```python
from build123d import *

# Parameters (mm, degrees)
SKETCH_2_R          = 1
CUT_EXTRUDE_1_DEPTH = 10
SKETCH_3_R          = 2.5
CUT_EXTRUDE_2_DEPTH = 2.5


with BuildPart() as part:
    # 草图1 → 旋转1 (revolve)
    with BuildSketch(Plane.XY, mode=Mode.PRIVATE) as revolve_1_sk:
        Polygon((0, 26), (3, 26), (3, 6), (9.5, 6), (10, 5.5), (10, 0), (3, 0), (3, 3), (0, 3), align=None)
    revolve(revolve_1_sk.sketch.rotate(Axis((0, 9.947317903, 0), (0, -1, 0)), 90), axis=Axis((0, 9.947317903, 0), (0, -1, 0)))

    # 草图2 → 切除-拉伸1 (cut)
    with BuildSketch(Plane(origin=(0, 6, 0), x_dir=(1, 0, 0), z_dir=(0, 1, 0))):
        with Locations(Location((0, 6, 0), (0, 0, 270))):
            Circle(SKETCH_2_R)
        with Locations(Location((6, 0, 0), (0, 0, 270))):
            Circle(SKETCH_2_R)
        with Locations(Location((0, -6, 0), (0, 0, 270))):
            Circle(SKETCH_2_R)
        with Locations(Location((-6, 0, 0), (0, 0, 270))):
            Circle(SKETCH_2_R)
    extrude(amount=-CUT_EXTRUDE_1_DEPTH, mode=Mode.SUBTRACT)

    # 草图3 → 切除-拉伸2 (cut)
    with BuildSketch(Plane(origin=(0, 6, 0), x_dir=(1, 0, 0), z_dir=(0, 1, 0))):
        with Locations(Location((0, 6, 0), (0, 0, 270))):
            Circle(SKETCH_3_R)
        with Locations(Location((6, 0, 0), (0, 0, 270))):
            Circle(SKETCH_3_R)
        with Locations(Location((0, -6, 0), (0, 0, 270))):
            Circle(SKETCH_3_R)
        with Locations(Location((-6, 0, 0), (0, 0, 270))):
            Circle(SKETCH_3_R)
    extrude(amount=-CUT_EXTRUDE_2_DEPTH, mode=Mode.SUBTRACT)


solid = part.part
```
Geometry: final body of the model. Coordinates: model frame, mm. A direction names the side the tool comes from. Round coordinates to 2 decimals unless told otherwise and drop trailing zeros. Order: outer loops, then holes, each group sorted by start corner. A loop starts at its lowest first (then second) coordinate and runs counter-clockwise, first axis right, second up. Notation, with made-up numbers: (21, -0.5) -> (71, -0.5) arc R16 ccw to (71, 12.5) -> close; hole circle Ø7 at (67, -20.75). An arc over 180 degrees is marked (long way). Use CSV: the item, a comma, the result in double quotes. Start each with the question number.
1) Set-up query: faces 4 (the face through (-0.6, 1.8, -6.8)), 5 (the face through (0, 3, 0)), 6 (the face through (0.751, 4.768, -3.615)). Return all of +Z, -Z, +X, -X, +Y, -Y with unobstructed straight access to the full face (end or side cutting, diameter ignored); none if empty.
2) Section C-C (y = 1.5). Return the cut outline in (x, z), and give its area (3 significant figures).
3) Section D-D (y = 20.75). Return the cut outline in (x, z), and give its area (3 significant figures).
4) Section A-A (x = 0). State how many separate pieces and enclosed holes the cut face has, and give its area (3 significant figures).
5) Draft query along X for faces 1 (the face through (-0.9, 15.86, 2.86)), 2 (the face through (0.751, 4.768, 8.385)), 3 (the face through (-2.4, 0, 2.1)). Return one class per face: +X half, -X half, draft (parallel to the pull), parting line (faces both ways), or undercut.
6) First-contact query: pin 1 Ø1.6 at (x, z) = (0, 6) entering from -Y; pin 2 Ø3 at (x, z) = (-0.5, 0) entering from -Y; pin 3 Ø1.5 at (x, z) = (1, 6) entering from +Y; pin 4 Ø12 at (y, z) = (19.5, -6.5) entering from +X. Flat tips, straight axial feed; report the tip coordinate or a pass-through.
7) Material intervals for line 1 along Z through (x, y) = (-2.25, 4.5); line 2 along Y through (x, z) = (3, 6.5); line 3 along Y through (x, z) = (-4.5, -1.5), sorted ascending. Write a range as from..to.
Returned:
1,face 4,"+Y, -Y"
1,face 5,"-Y"
1,face 6,"+Y"
2,outline,"circle Ø20 at (0, 0); hole circle Ø2 at (-6, 0); hole circle Ø6 at (0, 0); hole circle Ø2 at (0, -6); hole circle Ø2 at (0, 6); hole circle Ø2 at (6, 0)"
2,area,"273 mm²"
3,outline,"circle Ø6 at (0, 0)"
3,area,"28.3 mm²"
4,separate pieces,"3"
4,enclosed holes,"0"
4,area,"183 mm²"
5,face 1,"parting line"
5,face 2,"undercut"
5,face 3,"draft"
6,pin 1,"passes through"
6,pin 2,"stops at y = 3"
6,pin 3,"stops at y = 3.5"
6,pin 4,"stops at x = 2.96"
7,line 1,"z = -9.74..-7.09, -4.91..4.91, 7.09..9.74"
7,line 2,"y = 0..6"
7,line 3,"y = 0..3.5"
